Verification items for the finished model (mm, model axes). A direction names the side the tool comes from. Round coordinates to 2 decimals unless told otherwise and drop trailing zeros. Loops run counter-clockwise (first coordinate to the right, second up) from the corner with the lowest first, then second, coordinate; pieces in that order, holes last. Notation, with made-up numbers: (51.25, 13) -> (109.25, 13) arc R17 cw to (109.25, 28) -> close; hole circle Ø10 at (83, 77.25). An arc over 180 degrees is marked (long way). Use CSV: the item, a comma, the result in double quotes. Start each with the question number.
```python
from build123d import *

# Parameters (mm, degrees)
F1_DEPTH  = 40
F2_R      = 2
F3_DEPTH  = 80.001
F4_R      = 2
F6_W      = 20.5
F6_H      = 12
F7_DEPTH  = 10.501
F9_DEPTH  = 4.5
F10_R     = 3.25
F11_DEPTH = 22.501


# Not quite as in the source:
# - a pattern or mirror of a feature is missing from the dataset's text; its kind, count and spacing are read off the source's solid


with BuildPart() as f1:
    # F0 (on Right) → F1 (new body, symmetric)
    with BuildSketch(Plane.YZ):
        with BuildLine():
            Line((-17.5, 10), (-17.5, 0))
            Line((-17.5, 0), (12.5, 0))
            Line((12.5, 0), (12.5, 12.5))
            ThreePointArc((12.5, 12.5), (16.0355339059, 21.0355339059), (7.5, 17.5))
            Line((7.5, 17.5), (7.5, 10))
            Line((7.5, 10), (-17.5, 10))
        make_face()
    extrude(amount=F1_DEPTH, both=True)

    # F2 (on face) → F3 (cut, through all)
    with BuildSketch(Plane.YZ.offset(40)):
        with Locations((12.5, 17.5)):
            Circle(F2_R)
    extrude(amount=-F3_DEPTH, mode=Mode.SUBTRACT)

    # F4
    f4_edges = [f1.edges().sort_by_distance(p)[0] for p in [
        (0, 7.5, 10),
    ]]
    fillet(f4_edges, radius=F4_R)

    # F6 (on offset) → F7 (cut, through all)
    with BuildSketch(Plane.XY.offset(12)):
        with Locations((20, 13.5)):
            Rectangle(F6_W, F6_H)
    f7 = extrude(amount=F7_DEPTH, mode=Mode.SUBTRACT)

    # F7_copies: F7 across plane
    add(f7.mirror(Plane(origin=(0, 0, 0), x_dir=(0, 0, -1), z_dir=(-1, 0, 0))), mode=Mode.SUBTRACT)

    # F8 (on face) → F9 (cut)
    with BuildSketch(Plane.XY.offset(10)):
        Polygon((-3.0310889132, -5.25), (3.0310889132, -5.25), (6.0621778265, 0), (3.0310889132, 5.25), (-3.0310889132, 5.25), (-6.0621778265, 0), align=None)
    extrude(amount=-F9_DEPTH, mode=Mode.SUBTRACT)

    # F10 (on face) → F11 (cut, through all)
    with BuildSketch(Plane(origin=(0, 0, 0), x_dir=(1, 0, 0), z_dir=(0, 0, -1))):
        Circle(F10_R)
    extrude(amount=-F11_DEPTH, mode=Mode.SUBTRACT)


solid = f1.part
```
Q1. Depth check by flat-ended pin: pin 1 Ø5 at (x, y) = (0, -1) entering from +Z; pin 2 Ø5.5 at (x, y) = (-22.5, 10) entering from +Z; pin 3 Ø1.6 at (x, z) = (36.5, 15) entering from -Y; pin 4 Ø3.5 at (y, z) = (12.5, 17.5) entering from +X. Enter the tip coordinate at first touch or a pass-through.
Q2. Tool access check on faces 1 (the face through (1, 12.5, 6)), 2 (the face through (4.568, 2.588, 7.781)), 3 (the face through (35, 7.5, 15)), 4 (the face through (-9.75, 10, 17)). Record the directions out of +Z, -Z, +X, -X, +Y, -Y that give a thin tool (end or side, any length) a straight path to the whole face; none if there is none.
Q3. Cross-section at B-B (z = 7). Record the boundary of the cut face in (x, y), and give its area (3 significant figures).
Q4. Release check for a two-part mould opening along X. For faces 5 (the face through (4.525, -2.662, 7.781)), 6 (the face through (35.193, 12.24, 19.483)), 7 (the face through (3, 2, 5.5)) record: +X half, -X half, draft (parallel to the pull), parting line (faces both ways), or undercut.
Q5. Thickness scan on L1, parallel to Z at x = -10, y = 0; L2, parallel to X at y = 2.5, z = 1; L3, parallel to Z at x = -17.5, y = 11. Record the ranges inside material, lowest first. Write a range as from..to.
Q6. Cross-section at C-C (x = 8.5). Record the boundary of the cut face in (y, z).
Q7. Cross-section at A-A (x = 0). Record the boundary of the cut face in (y, z).
Answer list:
1,pin 1,"stops at z = 5.5"
1,pin 2,"stops at z = 12"
1,pin 3,"stops at y = 7.5"
1,pin 4,"passes through"
2,face 1,"-Z, +X, -X, +Y"
2,face 2,"+Z"
2,face 3,"+Z, +X, -X, -Y"
2,face 4,"+Z, +Y, -Y"
3,outline,"(-40, -17.5) -> (40, -17.5) -> (40, 12.5) -> (-40, 12.5) -> close; hole (-6.06, 0) -> (-3.03, -5.25) -> (3.03, -5.25) -> (6.06, 0) -> (3.03, 5.25) -> (-3.03, 5.25) -> close"
3,area,"2,300 mm2"
4,face 5,"undercut"
4,face 6,"draft"
4,face 7,"undercut"
5,L1,"z = 0..10"
5,L2,"x = -40..-2.08, 2.08..40"
5,L3,"z = 0..12"
6,outline,"(-17.5, 0) -> (12.5, 0) -> (12.5, 12.5) arc R5 ccw (long way) to (7.5, 17.5) -> (7.5, 12) arc R2 cw to (5.5, 10) -> (-17.5, 10) -> close; hole circle Ø4 at (12.5, 17.5)"
7,outline,"(-17.5, 0) -> (-3.25, 0) -> (-3.25, 5.5) -> (-5.25, 5.5) -> (-5.25, 10) -> (-17.5, 10) -> close; (3.25, 0) -> (12.5, 0) -> (12.5, 12.5) arc R5 ccw (long way) to (7.5, 17.5) -> (7.5, 12) arc R2 cw to (5.5, 10) -> (5.25, 10) -> (5.25, 5.5) -> (3.25, 5.5) -> close; hole circle Ø4 at (12.5, 17.5)"
